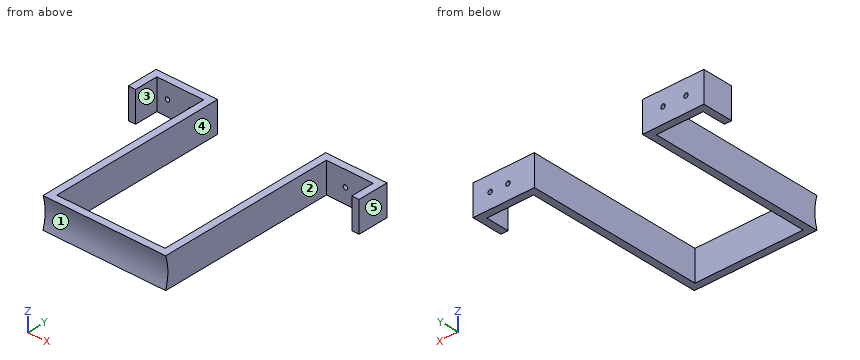
Autodesk Fusion 360 part; units mm, degrees
sketch "Sketch1" plane through (0, 0, 0) normal (0, 0, 1) x (1, 0, 0)
  line L0 (0, 0) -> (101.6, 0)
  line L1 (101.6, 0) -> (101.6, 6)
  line L2 (101.6, 6) -> (0, 6)
  line L3 (0, 6) -> (0, 0)
  dimension "d1" = 101.6
  dimension "d2" = 6
extrude "Extrude1" add sketch "Sketch1" along normal blind 25.4
sketch "Sketch2" plane through (0, 0, 25.4) normal (0, 0, 1) x (-1, 0, 0)
  line L0 (0, -6) -> (0, 0)
  line L1 (0, 0) -> (-101.6, 0)
  line L2 (-101.6, 0) -> (-101.6, -6)
  line L3 (-101.6, -6) -> (0, -6)
  line L4 (-101.6, 0) -> (-95.6, 0)
  line L5 (-95.6, 0) -> (-95.6, -152.4)
  line L6 (-95.6, -152.4) -> (-101.6, -152.4)
  line L7 (-101.6, -152.4) -> (-101.6, 0)
  dimension "d5" = 152.4
  dimension "d6" = 6
extrude "Extrude2" add sketch "Sketch2" against normal blind 25.4 contours L3 L5 L6 L7
sketch "Sketch3" plane through (0, 0, 25.4) normal (0, 0, 1) x (-1, 0, 0)
  line L0 (0, -6) -> (0, 0)
  line L1 (0, 0) -> (-101.6, 0)
  line L2 (-101.6, 0) -> (-101.6, -152.4)
  line L3 (-101.6, -152.4) -> (-95.6, -152.4)
  line L4 (-95.6, -152.4) -> (-95.6, -6)
  line L5 (-95.6, -6) -> (0, -6)
  line L6 (0, 0) -> (-6, 0)
  line L7 (-6, 0) -> (-6, -152.4)
  line L8 (-6, -152.4) -> (0, -152.4)
  line L9 (0, -152.4) -> (0, 0)
  dimension "d9" = 152.4
  dimension "d10" = 6
extrude "Extrude3" add sketch "Sketch3" against normal blind 25.4 contours L5 L7 L8 L9
sketch "Sketch4" plane through (101.6, 0, 0) normal (1, 0, 0) x (0, 1, 0)
  line L0 (0, 0) -> (152.4, 0)
  line L1 (152.4, 0) -> (152.4, 25.4)
  line L2 (152.4, 25.4) -> (0, 25.4)
  line L3 (0, 25.4) -> (0, 0)
  circle A0 centre (-39.719, 12.7) radius 41.7
  dimension "d13" = 83.4
extrude "Extrude4" cut sketch "Sketch4" against normal blind 101.6 contours L3 A0 picked at (0.3655, 9.8525)
sketch "Sketch5" plane through (0, 0, 25.4) normal (0, 0, 1) x (-1, 0, 0)
  line L0 (0, -152.4) -> (0, 0)
  line L1 (0, 0) -> (-101.6, 0)
  line L2 (-101.6, 0) -> (-101.6, -152.4)
  line L3 (-101.6, -152.4) -> (-95.6, -152.4)
  line L4 (-95.6, -152.4) -> (-95.6, -6)
  line L5 (-95.6, -6) -> (-6, -6)
  line L6 (-6, -6) -> (-6, -152.4)
  line L7 (-6, -152.4) -> (0, -152.4)
  line L8 (-6, -152.4) -> (44.8, -152.4)
  line L9 (44.8, -152.4) -> (44.8, -146.4)
  line L10 (44.8, -146.4) -> (-6, -146.4)
  line L11 (-6, -146.4) -> (-6, -152.4)
  dimension "d16" = 50.8
  dimension "d17" = 6
extrude "Extrude5" add sketch "Sketch5" against normal blind 25.4 contours L0 L8 L9 L10
sketch "Sketch6" plane through (0, 0, 25.4) normal (0, 0, 1) x (-1, 0, 0)
  line L0 (0, -146.4) -> (0, 0)
  line L1 (0, 0) -> (-101.6, 0)
  line L2 (-101.6, 0) -> (-101.6, -152.4)
  line L3 (-101.6, -152.4) -> (-95.6, -152.4)
  line L4 (-95.6, -152.4) -> (-95.6, -6)
  line L5 (-95.6, -6) -> (-6, -6)
  line L6 (-6, -6) -> (-6, -152.4)
  line L7 (-6, -152.4) -> (44.8, -152.4)
  line L8 (44.8, -152.4) -> (44.8, -146.4)
  line L9 (44.8, -146.4) -> (0, -146.4)
  line L10 (44.8, -152.4) -> (38.8, -152.4)
  line L11 (38.8, -152.4) -> (38.8, -127)
  line L12 (38.8, -127) -> (44.8, -127)
  line L13 (44.8, -127) -> (44.8, -152.4)
  dimension "d20" = 25.4
  dimension "d21" = 6
extrude "Extrude6" add sketch "Sketch6" against normal blind 25.4 contours L9 L11 L12 L13
sketch "Sketch7" plane through (0, 0, 25.4) normal (0, 0, 1) x (-1, 0, 0)
  line L0 (0, -146.4) -> (0, 0)
  line L1 (0, 0) -> (-101.6, 0)
  line L2 (-101.6, 0) -> (-101.6, -152.4)
  line L3 (-101.6, -152.4) -> (-95.6, -152.4)
  line L4 (-95.6, -152.4) -> (-95.6, -6)
  line L5 (-95.6, -6) -> (-6, -6)
  line L6 (-6, -6) -> (-6, -152.4)
  line L7 (-6, -152.4) -> (44.8, -152.4)
  line L8 (44.8, -152.4) -> (44.8, -127)
  line L9 (44.8, -127) -> (38.8, -127)
  line L10 (38.8, -127) -> (38.8, -146.4)
  line L11 (38.8, -146.4) -> (0, -146.4)
  line L12 (-95.6, -152.4) -> (-146.4, -152.4)
  line L13 (-146.4, -152.4) -> (-146.4, -146.4)
  line L14 (-146.4, -146.4) -> (-95.6, -146.4)
  line L15 (-95.6, -146.4) -> (-95.6, -152.4)
  dimension "d24" = 50.8
  dimension "d25" = 6
extrude "Extrude7" add sketch "Sketch7" against normal blind 25.4 contours L2 L12 L13 L14
sketch "Sketch8" plane through (0, 0, 25.4) normal (0, 0, 1) x (-1, 0, 0)
  line L0 (0, -146.4) -> (0, 0)
  line L1 (0, 0) -> (-101.6, 0)
  line L2 (-101.6, 0) -> (-101.6, -146.4)
  line L3 (-101.6, -146.4) -> (-146.4, -146.4)
  line L4 (-146.4, -146.4) -> (-146.4, -152.4)
  line L5 (-146.4, -152.4) -> (-95.6, -152.4)
  line L6 (-95.6, -152.4) -> (-95.6, -6)
  line L7 (-95.6, -6) -> (-6, -6)
  line L8 (-6, -6) -> (-6, -152.4)
  line L9 (-6, -152.4) -> (44.8, -152.4)
  line L10 (44.8, -152.4) -> (44.8, -127)
  line L11 (44.8, -127) -> (38.8, -127)
  line L12 (38.8, -127) -> (38.8, -146.4)
  line L13 (38.8, -146.4) -> (0, -146.4)
  line L14 (-146.4, -152.4) -> (-140.4, -152.4)
  line L15 (-140.4, -152.4) -> (-140.4, -127)
  line L16 (-140.4, -127) -> (-146.4, -127)
  line L17 (-146.4, -127) -> (-146.4, -152.4)
  dimension "d28" = 25.4
  dimension "d29" = 6
extrude "Extrude8" add sketch "Sketch8" against normal blind 25.4 contours L3 L15 L16 L17
sketch "Sketch9" plane through (0, 152.4, 0) normal (0, 1, 0) x (-1, 0, 0)
  line L0 (-95.6, 25.4) -> (-146.4, 25.4)
  line L1 (-146.4, 25.4) -> (-146.4, 0)
  line L2 (-146.4, 0) -> (-95.6, 0)
  line L3 (-95.6, 0) -> (-95.6, 25.4)
  circle A0 centre (-132.2412, 12.6561) radius 1.8288
  circle A1 centre (-112.7392, 12.6561) radius 1.8288
  dimension "d32" = 3.6576
  dimension "d33" = 3.6576
extrude "Extrude9" cut sketch "Sketch9" against normal blind 25 contours A0
sketch "Sketch10" plane through (0, 152.4, 0) normal (0, 1, 0) x (-1, 0, 0)
  circle A0 centre (-132.2412, 12.6561) radius 1.8288
  line L0 (-95.6, 25.4) -> (-146.4, 25.4)
  line L1 (-146.4, 25.4) -> (-146.4, 0)
  line L2 (-146.4, 0) -> (-95.6, 0)
  line L3 (-95.6, 0) -> (-95.6, 25.4)
  circle A1 centre (-117.3996, 12.4204) radius 1.8288
  dimension "d36" = 3.6576
extrude "Extrude10" cut sketch "Sketch10" against normal blind 30 contours A1
sketch "Sketch11" plane through (0, 152.4, 0) normal (0, 1, 0) x (-1, 0, 0)
  line L0 (44.8, 25.4) -> (-6, 25.4)
  line L1 (-6, 25.4) -> (-6, 0)
  line L2 (-6, 0) -> (44.8, 0)
  line L3 (44.8, 0) -> (44.8, 25.4)
  circle A0 centre (29.9851, 12.7) radius 1.8288
  dimension "d39" = 3.6576
extrude "Extrude11" cut sketch "Sketch11" against normal blind 20 contours A0
sketch "Sketch12" plane through (0, 152.4, 0) normal (0, 1, 0) x (-1, 0, 0)
  circle A0 centre (29.9851, 12.7) radius 1.8288
  line L0 (44.8, 25.4) -> (-6, 25.4)
  line L1 (-6, 25.4) -> (-6, 0)
  line L2 (-6, 0) -> (44.8, 0)
  line L3 (44.8, 0) -> (44.8, 25.4)
  circle A1 centre (10.9831, 12.9818) radius 1.8288
  dimension "d42" = 3.6576
extrude "Extrude12" cut sketch "Sketch12" against normal blind 30 contours A1
sketch "Sketch13" plane through (0, 0, 25.4) normal (0, 0, 1) x (-1, 0, 0)
  line L0 (0, -146.4) -> (0, 0)
  line L1 (0, 0) -> (-101.6, 0)
  line L2 (-101.6, 0) -> (-101.6, -146.4)
  line L3 (-101.6, -146.4) -> (-140.4, -146.4)
  line L4 (-140.4, -146.4) -> (-140.4, -127)
  line L5 (-140.4, -127) -> (-146.4, -127)
  line L6 (-146.4, -127) -> (-146.4, -152.4)
  line L7 (-146.4, -152.4) -> (-95.6, -152.4)
  line L8 (-95.6, -152.4) -> (-95.6, -6)
  line L9 (-95.6, -6) -> (-6, -6)
  line L10 (-6, -6) -> (-6, -152.4)
  line L11 (-6, -152.4) -> (44.8, -152.4)
  line L12 (44.8, -152.4) -> (44.8, -127)
  line L13 (44.8, -127) -> (38.8, -127)
  line L14 (38.8, -127) -> (38.8, -146.4)
  line L15 (38.8, -146.4) -> (0, -146.4)
Check sheet for the modelled part. Datum: model origin and axes. Units: mm. Face numbers are marked on the shaded views. A direction names the side the tool comes from. Coordinates: 2 decimals unless noted, no trailing zeros. Order: outer loops, then holes, each group sorted by start corner. A loop starts at its lowest first (then second) coordinate and runs counter-clockwise, first axis right, second up. Notation, with made-up numbers: (71, 60.25) -> (112, 60.25) arc R19 ccw to (112, 71.25) -> close; hole circle Ø3 at (-24, 65). An arc over 180 degrees is marked (long way). Write item = value, one per line. Start each with the question number.
1) Access from +Z, -Z, +X, -X, +Y, -Y to the whole of each face (thin tool, end or side, straight path). Record for the marked faces 3, 4 and 5.
2) Cross-section at A-A (y = 113). Enter the section's corners in (x, z).
3) Cross-section at D-D (x = 79). Enter the section's corners in (y, z), then the cut area to 3 significant figures.
4) Cross-section at B-B (z = 22.5). Enter the section's corners in (x, y).
5) Go/stop test with flat-tipped pins: P1, Ø12.5, axis at x = 118.5, z = 15.5, coming from the -Y side; P2, Ø5, axis at x = 83, z = 3, coming from the +Y side; P3, Ø3, axis at y = 84, z = 15, coming from the -X side; P4, Ø4, axis at x = -10.98, z = 12.98, coming from the +Y side. Record where each tip stops, or that it passes through.
6) Cross-section at C-C (x = -25). Enter the section's corners in (y, z).
7) Mould release check, pull along Z, two halves, no side actions. Record for the marked faces 1 and 2: +Z half, -Z half, draft (parallel to the pull), parting line (faces both ways), or undercut.
8) Material ranges on L1, parallel to X at y = 43.5, z = 12.75; L2, parallel to X at y = 135.5, z = 12.25; L3, parallel to Y at x = 111, z = 16.75, recorded low to high.
Ans:
q1.face_3 = +Z, -Z, -Y
q1.face_4 = +Z, -Z, +Y
q1.face_5 = +Z, -Z, +X, +Y, -Y
q2.outline = (0, 0) -> (6, 0) -> (6, 25.4) -> (0, 25.4) -> close; (95.6, 0) -> (101.6, 0) -> (101.6, 25.4) -> (95.6, 25.4) -> close
q3.outline = (0, 0) -> (6, 0) -> (6, 25.4) -> (0, 25.4) arc R41.7 cw to start
q3.area = 119 mm²
q4.outline = (-44.8, 127) -> (-38.8, 127) -> (-38.8, 146.4) -> (0, 146.4) -> (0, 0.81) -> (101.6, 0.81) -> (101.6, 146.4) -> (140.4, 146.4) -> (140.4, 127) -> (146.4, 127) -> (146.4, 152.4) -> (95.6, 152.4) -> (95.6, 6) -> (6, 6) -> (6, 152.4) -> (-44.8, 152.4) -> close
q5.P1 = 146.4
q5.P2 = 6
q5.P3 = 0
q5.P4 = 152.4
q6.outline = (146.4, 0) -> (152.4, 0) -> (152.4, 25.4) -> (146.4, 25.4) -> close
q7.face_1 = undercut
q7.face_2 = draft
q8.L1 = 0 to 6, 95.6 to 101.6
q8.L2 = -44.8 to -38.8, 0 to 6, 95.6 to 101.6, 140.4 to 146.4
q8.L3 = 146.4 to 152.4
